```python
from build123d import *

# Parameters (mm, degrees)
SKETCH1_R           = 85.2
SKETCH1_R_2         = 5
BOSS_EXTRUDE1_DEPTH = 1.5875


with BuildPart() as part:
    # Sketch1 → Boss-Extrude1 (new body)
    with BuildSketch(Plane(origin=(0, 0, 0), x_dir=(1, 0, 0), z_dir=(0, 1, 0))):
        Circle(SKETCH1_R)
        Circle(SKETCH1_R_2, mode=Mode.SUBTRACT)
        with BuildLine():
            ThreePointArc((70.961061147, 17.132653061), (67.785714286, 27.094223347), (63.219854476, 36.5))
            ThreePointArc((63.219854476, 36.5), (59.121778265, 37.598076211), (58.023702054, 33.5))
            ThreePointArc((58.023702054, 33.5), (62.214285714, 24.86730088), (65.128645162, 15.724489796))
            ThreePointArc((65.128645162, 15.724489796), (68.748934787, 13.512363436), (70.961061147, 17.132653061))
        make_face(mode=Mode.SUBTRACT)
        with BuildLine():
            ThreePointArc((20.643217788, 70.020408163), (10.428571429, 72.251262259), (0, 73))
            ThreePointArc((0, 73), (-3, 70), (0, 67))
            ThreePointArc((0, 67), (9.571428571, 66.312802347), (18.946514956, 64.265306122))
            ThreePointArc((18.946514956, 64.265306122), (22.672417393, 66.294505727), (20.643217788, 70.020408163))
        make_face(mode=Mode.SUBTRACT)
        with BuildLine():
            ThreePointArc((50.317843359, -52.887755102), (57.357142857, -45.157038912), (63.219854476, -36.5))
            ThreePointArc((63.219854476, -36.5), (62.121778265, -32.401923789), (58.023702054, -33.5))
            ThreePointArc((58.023702054, -33.5), (52.642857143, -41.445501467), (46.182130206, -48.540816327))
            ThreePointArc((46.182130206, -48.540816327), (46.076517395, -52.782142291), (50.317843359, -52.887755102))
        make_face(mode=Mode.SUBTRACT)
        with BuildLine():
            ThreePointArc((-20.643217788, -70.020408163), (-10.428571429, -72.251262259), (0, -73))
            ThreePointArc((0, -73), (3, -70), (0, -67))
            ThreePointArc((0, -67), (-9.571428571, -66.312802347), (-18.946514956, -64.265306122))
            ThreePointArc((-18.946514956, -64.265306122), (-22.672417393, -66.294505727), (-20.643217788, -70.020408163))
        make_face(mode=Mode.SUBTRACT)
        with BuildLine():
            ThreePointArc((-70.961061147, -17.132653061), (-67.785714286, -27.094223347), (-63.219854476, -36.5))
            ThreePointArc((-63.219854476, -36.5), (-59.121778265, -37.598076211), (-58.023702054, -33.5))
            ThreePointArc((-58.023702054, -33.5), (-62.214285714, -24.86730088), (-65.128645162, -15.724489796))
            ThreePointArc((-65.128645162, -15.724489796), (-68.748934787, -13.512363436), (-70.961061147, -17.132653061))
        make_face(mode=Mode.SUBTRACT)
        with BuildLine():
            ThreePointArc((-50.317843359, 52.887755102), (-57.357142857, 45.157038912), (-63.219854476, 36.5))
            ThreePointArc((-63.219854476, 36.5), (-62.121778265, 32.401923789), (-58.023702054, 33.5))
            ThreePointArc((-58.023702054, 33.5), (-52.642857143, 41.445501467), (-46.182130206, 48.540816327))
            ThreePointArc((-46.182130206, 48.540816327), (-46.076517395, 52.782142291), (-50.317843359, 52.887755102))
        make_face(mode=Mode.SUBTRACT)
    extrude(amount=BOSS_EXTRUDE1_DEPTH)


solid = part.part
```
Geometry check sheet. Reference: the model listing, model coordinates, mm. A direction names the side the tool comes from. Round coordinates to 2 decimals unless told otherwise and drop trailing zeros. Order: outer loops, then holes, each group sorted by start corner. A loop starts at its lowest first (then second) coordinate and runs counter-clockwise, first axis right, second up. Notation, with made-up numbers: (-10.75, 40.25) -> (28.25, 40.25) arc R23 ccw to (28.25, 54.25) -> close; hole circle Ø7 at (55, -1). An arc over 180 degrees is marked (long way). Return JSON: item names as keys, results as strings. Group by question number.
Q1. Tool access check on faces 4 (the flat face through (18, 1.588, -1)), 5 (the cylindrical face through (57.27, 0.78, 45.27)). Record the directions out of +Z, -Z, +X, -X, +Y, -Y that give a thin tool (end or side, any length) a straight path to the whole face; none if there is none.
Q2. Section check B-B, the plane y = 1.1. Record the boundary of the cut face in (x, z).
Q3. Section check D-D, the plane x = -42. Record the boundary of the cut face in (y, z), plus the area to 3 significant figures.
Q4. Material ranges on probe 1 along X at (y, z) = (1.1, 0); probe 2 along Z at (x, y) = (4, 1.1); probe 3 along X at (y, z) = (0.1, 35), recorded low to high. Write a range as from..to.
Q5. Section check C-C, the plane x = -15. Record the boundary of the cut face in (y, z), plus the area to 3 significant figures.
Q6. Release check for a two-part mould opening along Z. For faces 1 (the flat face through (18, 0, -1)), 2 (the cylindrical face through (81.266, 0.783, -25.592)), 3 (the cylindrical face through (46, 0.8, 52.7)) record: released by +Z, released by -Z, zero draft, split by the parting line, or undercut.
Q7. Section check A-A, the plane z = 0. Record the boundary of the cut face in (x, y).
Numbers:
{
 "1": {"face 4": "+Z, -Z, +X, -X, +Y", "face 5": "+Y, -Y"},
 "2": {"outline": "circle Ø170.4 at (0, 0); hole (-70.96, 17.13) arc R3 ccw to (-65.13, 15.72) arc R67 cw to (-58.02, 33.5) arc R3 ccw to (-63.22, 36.5) arc R73 ccw to start; hole (-63.22, -36.5) arc R73 ccw to (-50.32, -52.89) arc R3 ccw to (-46.18, -48.54) arc R67 cw to (-58.02, -33.5) arc R3 ccw to start; hole (-20.64, 70.02) arc R3 ccw to (-18.95, 64.27) arc R67 cw to (0, 67) arc R3 ccw to (0, 73) arc R73 ccw to start; hole circle Ø10 at (0, 0); hole (0, -73) arc R73 ccw to (20.64, -70.02) arc R3 ccw to (18.95, -64.27) arc R67 cw to (0, -67) arc R3 ccw to start; hole (46.18, 48.54) arc R67 cw to (58.02, 33.5) arc R3 ccw to (63.22, 36.5) arc R73 ccw to (50.32, 52.89) arc R3 ccw to start; hole (58.02, -33.5) arc R3 ccw to (63.22, -36.5) arc R73 ccw to (70.96, -17.13) arc R3 ccw to (65.13, -15.72) arc R67 cw to start"},
 "3": {"outline": "(0, -74.13) -> (1.59, -74.13) -> (1.59, 74.13) -> (0, 74.13) -> close", "area": "235 mm^2"},
 "4": {"probe 1": "-85.2..-5, 5..85.2", "probe 2": "-85.11..-72.89, -66.88..-3, 3..85.11", "probe 3": "-77.68..-64.06, -57.62..57.13, 63.62..77.68"},
 "5": {"outline": "(0, -83.87) -> (1.59, -83.87) -> (1.59, 65.3) -> (0, 65.3) -> close; (0, 71.44) -> (1.59, 71.44) -> (1.59, 83.87) -> (0, 83.87) -> close", "area": "257 mm^2"},
 "6": {"face 1": "zero draft", "face 2": "split by the parting line", "face 3": "undercut"},
 "7": {"outline": "(-85.2, 0) -> (-5, 0) -> (-5, 1.59) -> (-85.2, 1.59) -> close; (5, 0) -> (85.2, 0) -> (85.2, 1.59) -> (5, 1.59) -> close"}
}
